Print and shaded views of the part. All mm, measured from the part's lowest x, y and z. A direction names the side the tool comes from. Coordinates: 2 decimals unless noted, no trailing zeros. Loops run counter-clockwise (first coordinate to the right, second up) from the corner with the lowest first, then second, coordinate; pieces in that order, holes last. Notation, with made-up numbers: M 79.25,77.5 L 123.25,77.5 A35 cw 123.25,114.5 Z; hole C 21,11 d6. An arc over 180 degrees is marked long. Answer as a JSON object with one key per item and string values. Group by question number.
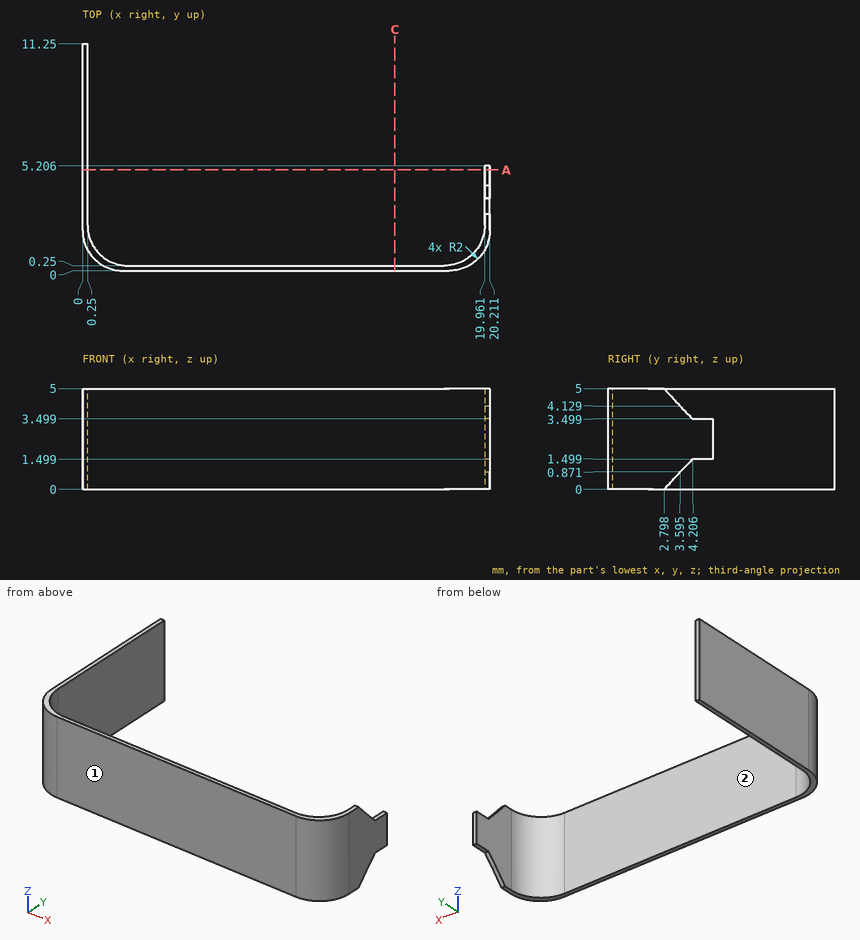
Item 1: Tool access for the marked faces 1 and 2: list every direction of +Z, -Z, +X, -X, +Y, -Y with a clear straight run to the whole face (end or side of a thin tool).
Item 2: Pin check, flat tip, straight feed: pin 1 (4 mm diameter, centred on x = 11, y = 1.5, fed in from -Z). Stop position of the tip, or through.
Item 3: Slice it at A-A, the plane y = 5. Write the cut outline in (x, z).
Item 4: Drill centre lines: L1, parallel to Y at x = 7, z = 4; L2, parallel to X at y = 2.5, z = 0.45. Where is each one in solid material? Low to high. Write a range as from..to.
Item 5: Slice it at C-C, the plane x = 15.5. Write the cut outline in (y, z).
Computed:
{
 "1": {"face 1": "+Z, -Z, +X, -X, -Y", "face 2": "+Z, -Z, +Y"},
 "2": {"pin 1": "z = 0"},
 "3": {"outline": "M 0,0 L 0.25,0 L 0.25,5 L 0,5 Z; M 19.96,1.5 L 20.21,1.5 L 20.21,3.5 L 19.96,3.5 Z"},
 "4": {"L1": "0..0.25", "L2": "0..0.25, 19.96..20.21"},
 "5": {"outline": "M 0,0 L 0.25,0 L 0.25,5 L 0,5 Z"}
}
